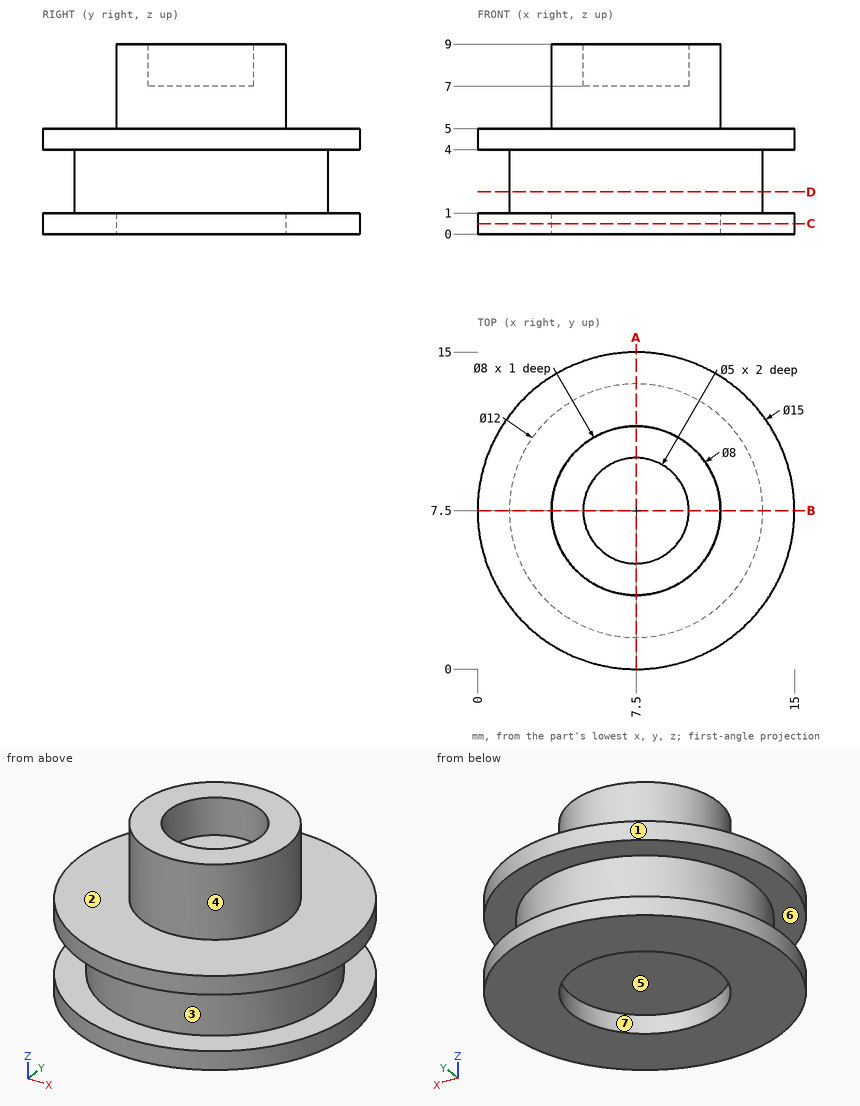
Print and shaded views of the part. All mm, measured from the part's lowest x, y and z. A direction names the side the tool comes from. Round coordinates to 2 decimals unless told otherwise and drop trailing zeros. Write each loop counter-clockwise with the first axis right and the second up, starting at its lowest first coordinate (ties: lowest second). Pieces come first, ordered by that corner, then holes.
Item 1: Cut at C-C, the plane z = 0.5. Give the cut face in (x, y), plus the area to 3 significant figures.
Results:
outline: circle Ø15 at (7.5, 7.5); hole circle Ø8 at (7.5, 7.5)
area: 126 mm2
Item 2: Which spindle directions (+Z, -Z, +X, -X, +Y, -Y) get a long thin tool onto all of the face, cutting with end or side? Do the marked faces 1, 2 and 3. Say none if no direction does.
Results:
face 1: +Z, -Z
face 2: +Z
face 3: none
Item 3: Cut at D-D, the plane z = 2. Give the cut face in (x, y).
Results:
outline: circle Ø12 at (7.5, 7.5)
Item 4: Probe L1, parallel to Z at x = 12, y = 3; L2, parallel to Z at x = 12.25, y = 7.75; L3, parallel to Y at x = 7.5, z = 0.35. List the from-to ranges inside material, lowest first.
Results:
L1: z = 0 to 1, 4 to 5
L2: z = 0 to 5
L3: y = 0 to 3.5, 11.5 to 15
Item 5: Drop flat-ended pins along their axis: pin 1 Ø3 at (x, y) = (5, 5.5) entering from -Z; pin 2 Ø4 at (x, y) = (4.5, 13) entering from +Z; pin 3 Ø6.5 at (x, y) = (7.5, 7.5) entering from -Z; pin 4 Ø2 at (x, z) = (11, 5.5) entering from +Y. Give the stop position or say it passes through.
Results:
pin 1: stops at z = 0
pin 2: stops at z = 5
pin 3: stops at z = 1
pin 4: stops at y = 14.52
Item 6: Two-plate mould, pull along X, no slides. Class the marked faces 4, 5, 6 and 7: +X half, -X half, draft (parallel to the pull), parting line (faces both ways), or undercut.
Results:
face 4: parting line
face 5: undercut
face 6: draft
face 7: undercut
Item 7: Cut at A-A, the plane x = 7.5. Give the cut face in (y, z), plus the area to 3 significant figures.
Results:
outline: (0, 0) - (3.5, 0) - (3.5, 1) - (11.5, 1) - (11.5, 0) - (15, 0) - (15, 1) - (13.5, 1) - (13.5, 4) - (15, 4) - (15, 5) - (11.5, 5) - (11.5, 9) - (10, 9) - (10, 7) - (5, 7) - (5, 9) - (3.5, 9) - (3.5, 5) - (0, 5) - (0, 4) - (1.5, 4) - (1.5, 1) - (0, 1) - close
area: 80.0 mm2
